Solid Edge part; units mm, degrees
sketch "Sketch1" plane through (0, 0, 0) normal (0, -1, 0) x (1, 0, 0)
  line L0 (30, 0) -> (65, 30)
  line L1 (65, 30) -> (90, 30)
  line L2 (90, 30) -> (90, 35)
  line L3 (90, 35) -> (56.9204, 35)
  line L4 (56.9204, 35) -> (0, 35)
  line L5 (0, 35) -> (0, 30)
  line L6 (0, 30) -> (23, 30)
  line L7 (23, 30) -> (23, 8)
  line L8 (23, 8) -> (0, 8)
  line L9 (0, 8) -> (0, 0)
  line L10 (0, 0) -> (30, 0)
  dimension "D1" = 23
extrude "Protrusion1" add sketch "Sketch1" against normal blind 50
mirror "Mirror1" about plane through (0, 25, 4) normal (-1, 0, 0) of "Protrusion1"
sketch "Sketch2" plane through (0, 0, 26) normal (0, -1, 0) x (1, 0, 0)
  line L0 (30, -16.6796) -> (54.1262, 4)
  line L1 (54.1262, 4) -> (30, 4)
  line L2 (30, 4) -> (30, -16.6796)
extrude "Cutout1" cut sketch "Sketch2" against normal through all
sketch "Sketch3" plane through (0, 25, 0) normal (0, 0, -1) x (1, 0, 0)
  circle A0 centre (-16, 21) radius 1.75
  circle A1 centre (16, 21) radius 1.75
  circle A2 centre (16, -21) radius 1.75
  circle A3 centre (-16, -21) radius 1.75
extrude "Cutout2" cut sketch "Sketch3" against normal up to next
sketch "Sketch4" plane through (0, 25, 8) normal (0, 0, 1) x (1, 0, 0)
  circle A0 centre (-16, -21) radius 3.75
  circle A1 centre (16, -21) radius 3.75
  circle A2 centre (-16, 21) radius 3.75
  circle A3 centre (16, 21) radius 3.75
extrude "Extrusionsausschnitt_4" cut sketch "Sketch4" against normal blind 4
mirror "Mirror2" about plane through (0, 0, 0) normal (1, 0, 0) of "Cutout1"
sketch "Sketch5" plane through (0, 25, 35) normal (0, 0, 1) x (-1, 0, 0)
  line L0 (-100, -40) -> (100, -40)
  line L1 (100, -40) -> (100, 40)
  line L2 (100, 40) -> (-100, 40)
  line L3 (-100, 40) -> (-100, -40)
  dimension "D1" = 100
  dimension "D2" = 100
extrude "Protrusion2" add sketch "Sketch5" against normal up to vertex (5 mm away)
sketch "Sketch6" plane through (0, 25, 35) normal (0, 0, 1) x (-1, 0, 0)
  circle A0 centre (-90, -32.5) radius 2.25
  circle A1 centre (-40, 32.5) radius 2.25
  circle A2 centre (-40, -32.5) radius 2.25
  circle A3 centre (40, 32.5) radius 2.25
  circle A4 centre (40, -32.5) radius 2.25
  circle A5 centre (90, -32.5) radius 2.25
  circle A6 centre (90, 32.5) radius 2.25
  circle A7 centre (-90, 32.5) radius 2.25
  dimension "D1" = 65
extrude "Cutout3" cut sketch "Sketch6" against normal up to next
chamfer "Fase_2" distance 0.5 angle 45 8 edges at (92.25, 57.5, 30) (92.25, -7.5, 30) (42.25, -7.5, 30) (-37.75, -7.5, 30) (-87.75, -7.5, 30) (-87.75, 57.5, 30) (-37.75, 57.5, 30) (42.25, 57.5, 30)
properties material "Nylon, allgemein"
Check sheet for the modelled part. Datum: model origin and axes. Units: mm. A direction names the side the tool comes from. Round coordinates to 2 decimals unless told otherwise and drop trailing zeros. Order: outer loops, then holes, each group sorted by start corner. A loop starts at its lowest first (then second) coordinate and runs counter-clockwise, first axis right, second up.
1) Go/stop test with flat-tipped pins: pin 1 Ø12 at (x, y) = (-45, 19) entering from -Z; pin 2 Ø2.5 at (x, y) = (40, -7.5) entering from -Z; pin 3 Ø1.5 at (x, y) = (-26.5, -1) entering from -Z; pin 4 Ø2 at (y, z) = (22.5, 11.5) entering from -X. Record where each tip stops, or that it passes through.
2) Section check B-B (x = -5). Record the boundary of the cut face in (y, z).
3) Scan lines: line 1 (X direction, y = -7.5, z = 33.45); line 2 (Y direction, x = 16, z = 3); line 3 (Y direction, x = -16, z = 6.8). Record each from-to range of solid material in increasing order.
4) Section check C-C (x = 90). Record the boundary of the cut face in (y, z), and give its area (4 significant figures).
5) Mould release check, pull along Y, two halves, no side actions. Record for faces 5 (the flat face through (23, 25, 19)), 6 (the cylindrical face through (87.854, -8.176, 32.782)), 7 (the cylindrical face through (-92.146, 56.824, 32.782)), 8 (the flat face through (1, 0, 5)): +Y half, -Y half, draft (parallel to the pull), parting line (faces both ways), or undercut.
6) Tool access check on faces 1 (the cylindrical face through (-16.81, 0.34, 6.03)), 2 (the cylindrical face through (40.29, 55.27, 32.78)), 3 (the flat face through (0, 25, 8)), 4 (the cylindrical face through (15.62, 47.71, 1.97)). Record the directions out of +Z, -Z, +X, -X, +Y, -Y that give a thin tool (end or side, any length) a straight path to the whole face; none if there is none.
7) Section check A-A (y = 4). Give the number of separate pieces and of enclosed holes in the cut face, and give its area (3 significant figures).
8) Section check D-D (y = 33.5). Record the boundary of the cut face in (x, z).
Result:
1. pin 1: stops at z = 7.71
1. pin 2: passes through
1. pin 3: stops at z = 30
1. pin 4: stops at x = -44.58
2. outline: (-15, 30) - (65, 30) - (65, 35) - (-15, 35) - close; (0, 0) - (50, 0) - (50, 8) - (0, 8) - close
3. line 1: x = -100 to -92.25, -87.75 to -42.25, -37.75 to 37.75, 42.25 to 87.75, 92.25 to 100
3. line 2: y = 0 to 2.25, 5.75 to 44.25, 47.75 to 50
3. line 3: y = 0 to 0.25, 7.75 to 42.25, 49.75 to 50
4. outline: (-15, 30) - (-10.25, 30) - (-9.75, 30.5) - (-9.75, 35) - (-15, 35) - close; (-5.25, 30.5) - (-4.75, 30) - (54.75, 30) - (55.25, 30.5) - (55.25, 35) - (-5.25, 35) - close; (59.75, 30.5) - (60.25, 30) - (65, 30) - (65, 35) - (59.75, 35) - close
4. area: 354.5 mm2
5. face 5: draft
5. face 6: undercut
5. face 7: undercut
5. face 8: -Y half
6. face 1: none
6. face 2: +Z, -Z
6. face 3: +Y, -Y
6. face 4: -Z
7. separate pieces: 2
7. enclosed holes: 2
7. area: 2,250 mm2
8. outline: (-100, 30) - (-65, 30) - (-30, 0) - (30, 0) - (65, 30) - (100, 30) - (100, 35) - (-100, 35) - close; hole (-54.13, 30) - (-30, 9.32) - (-30, 30) - close; hole (-23, 8) - (23, 8) - (23, 30) - (-23, 30) - close; hole (30, 9.32) - (54.13, 30) - (30, 30) - close
